Drawing for the job (mm, zero at the part's lowest x, y, z). Coordinates: 2 decimals unless noted, no trailing zeros. Write each loop counter-clockwise with the first axis right and the second up, starting at its lowest first coordinate (ties: lowest second). Pieces come first, ordered by that corner, then holes. Notation, with made-up numbers: (-39.75, 1) -> (-29.75, 1) arc R15 cw to (-29.75, 14) -> close; hole circle Ø11 at (49.5, 50). An arc over 180 degrees is marked (long way). Answer as CSV lines item,"result". Start each with the question number.
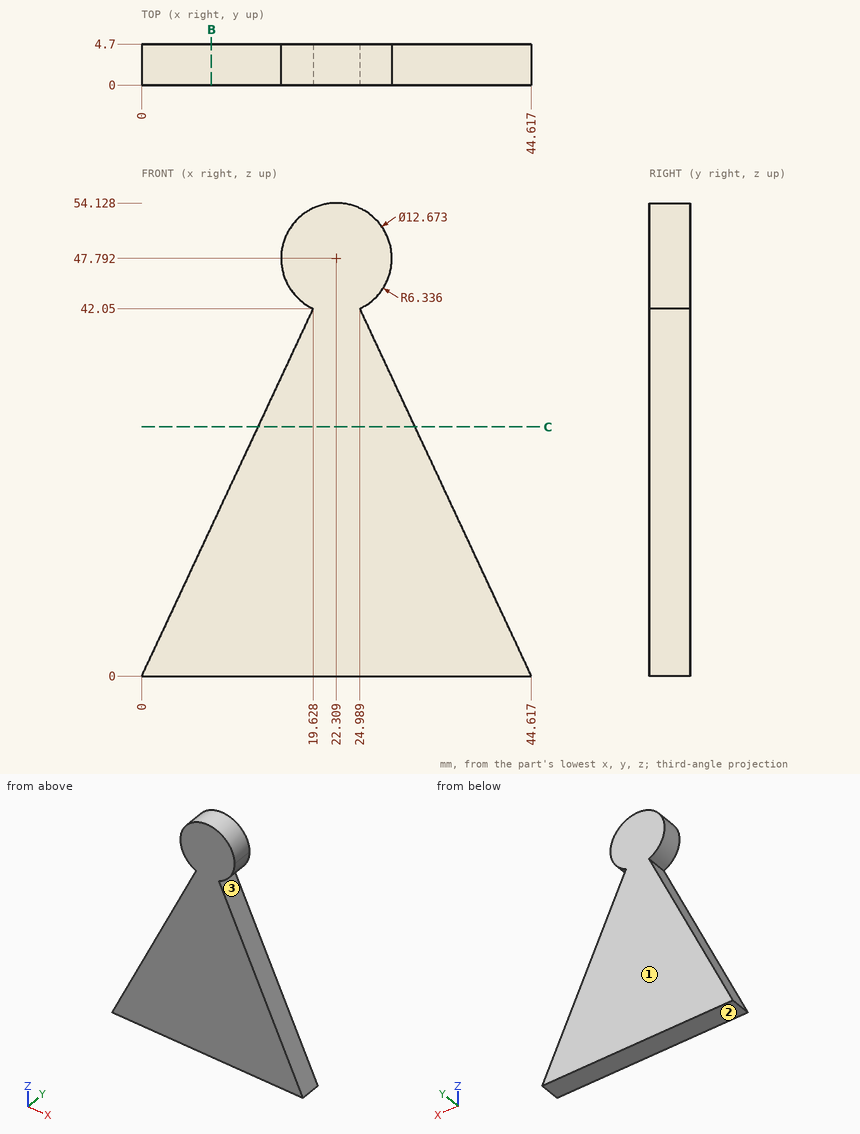
1. Flat gauge pins, fed straight in: P1, Ø2, axis at y = 2, z = 25, coming from the +X side (1 decimal); P2, Ø8, axis at x = 22, z = 41.5, coming from the -Y side. Where does each tip first touch, or does it go through?
2. Mould opens along Z. For the marked faces 1, 2 and 3 say: pulls with the +Z half, pulls with the -Z half, needs draft (parallel to the pull), parting line crosses it, or undercut.
3. Cut at B-B (x = 8). Give the cut face in (y, z).
4. Wall check: line 1 (Z direction, x = 28, y = 0.55) (1 decimal); line 2 (Z direction, x = 17.5, y = 4.2) (1 decimal); line 3 (Z direction, x = 22, y = 1.9). Give the ranges that are in metal, low to high.
5. Cut at C-C (z = 28.5). Give the cut face in (x, y).
Geometry check:
1,P1,"x = 33.4"
1,P2,"y = 0"
2,face 1,"needs draft"
2,face 2,"pulls with the -Z half"
2,face 3,"undercut"
3,outline,"(0, 0) -> (4.7, 0) -> (4.7, 17.14) -> (0, 17.14) -> close"
4,line 1,"0 to 35.6, 45 to 50.6"
4,line 2,"0 to 37.5, 43.7 to 51.9"
4,line 3,"0 to 54.12"
5,outline,"(13.3, 0) -> (31.31, 0) -> (31.31, 4.7) -> (13.3, 4.7) -> close"
